Here's how the part is built. I have some questions about the finished solid (model axes, mm). Face numbers are marked on the shaded views. Round coordinates to 2 decimals unless told otherwise and drop trailing zeros. Order: outer loops, then holes, each group sorted by start corner. A loop starts at its lowest first (then second) coordinate and runs counter-clockwise, first axis right, second up.
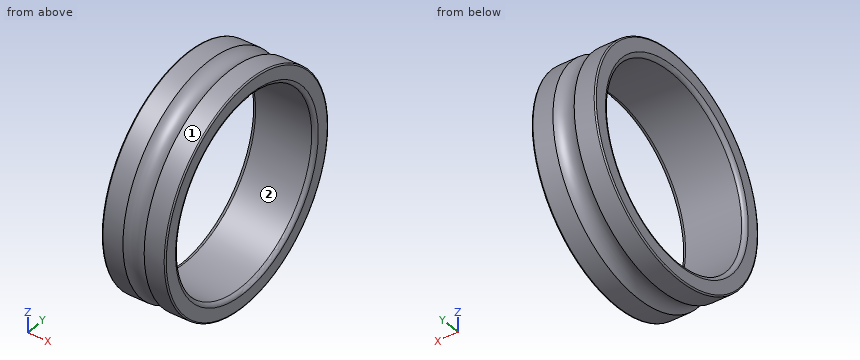
```python
from build123d import *


with BuildPart() as part:
    # 草图1 → 旋转1 (revolve)
    with BuildSketch(Plane.XY):
        with BuildLine():
            Line((0, 8.8), (0, 7.8))
            ThreePointArc((0, 7.8), (0.087867966, 7.587867966), (0.3, 7.5))
            Line((0.3, 7.5), (4.7, 7.5))
            ThreePointArc((4.7, 7.5), (4.912132034, 7.587867966), (5, 7.8))
            Line((5, 7.8), (5, 8.8))
            ThreePointArc((5, 8.8), (4.970710678, 8.870710678), (4.9, 8.9))
            Line((4.9, 8.9), (3.333540791, 8.9))
            ThreePointArc((3.333540791, 8.9), (2.5, 8.5595), (1.666459209, 8.9))
            Line((1.666459209, 8.9), (0.1, 8.9))
            ThreePointArc((0.1, 8.9), (0.029289322, 8.870710678), (0, 8.8))
        make_face()
    revolve(axis=Axis((50, 0, 0), (-1, 0, 0)))


solid = part.part
```
1. If we section it at A-A, the plane y = 0: Write out the boundary of the cut face in (x, z), and give its area (3 significant figures).
Evaluation:
outline: (0, -8.8) arc R0.1 ccw to (0.1, -8.9) - (1.67, -8.9) arc R1.19 cw to (3.33, -8.9) - (4.9, -8.9) arc R0.1 ccw to (5, -8.8) - (5, -7.8) arc R0.3 ccw to (4.7, -7.5) - (0.3, -7.5) arc R0.3 ccw to (0, -7.8) - close; (0, 7.8) arc R0.3 ccw to (0.3, 7.5) - (4.7, 7.5) arc R0.3 ccw to (5, 7.8) - (5, 8.8) arc R0.1 ccw to (4.9, 8.9) - (3.33, 8.9) arc R1.19 cw to (1.67, 8.9) - (0.1, 8.9) arc R0.1 ccw to (0, 8.8) - close
area: 13.1 mm2
2. If we section it at C-C, the plane x = 4: Write out the boundary of the cut face in (y, z).
Evaluation:
outline: circle Ø17.8 at (0, 0); hole circle Ø15 at (0, 0)
3. I'm going to push a flat-ended pin straight in: P1, Ø1, axis at x = 2.5, z = 5.5, coming from the -Y side. Where does the tip first touch, or does it pass through?
Evaluation:
P1: stops at y = -6.95
4. I need wall thicknesses on probe 1 along Z at (x, y) = (1.5, 0); probe 2 along Y at (x, z) = (1.9, 6.25). Which ranges of each line are inside material? Lowest first, please.
Evaluation:
probe 1: z = -8.9 to -7.5, 7.5 to 8.9
probe 2: y = -6.08 to -4.15, 4.15 to 6.08
5. If we mould it in two halves opening along Z, with no side actions, what happens to the marked faces 1 and 2? For each: released by +Z, released by -Z, zero draft, split by the parting line, or undercut.
Evaluation:
face 1: split by the parting line
face 2: undercut
